```python
from build123d import *

# Parameters (mm, degrees)
AUFSATZ_LINEAR_AUSTRAGEN1_DEPTH             = 21
AUFSATZ_LINEAR_AUSTRAGEN1_DEPTH_BACK        = 21
SCHNITT_LINEAR_AUSTRAGEN1_DEPTH             = 35
SKIZZE9_R                                   = 4
SCHNITT_LINEAR_AUSTRAGEN2_DEPTH             = 21
SCHNITT_LINEAR_AUSTRAGEN3_REACH             = 35.5
SKIZZE11_R                                  = 3
SCHNITT_LINEAR_AUSTRAGEN3_DIRECTION_2_REACH = 35.5


with BuildPart() as part:
    # Skizze3 → Aufsatz-Linear austragen1 (new body, two sides)
    with BuildSketch(Plane.XY) as aufsatz_linear_austragen1_sk:
        Polygon((0, 205), (33.5, 205), (33.5, 130), (11, 130), (11, 155), (0, 155), (-11, 155), (-11, 130), (-33.5, 130), (-33.5, 205), align=None)
    extrude(amount=AUFSATZ_LINEAR_AUSTRAGEN1_DEPTH)
    extrude(aufsatz_linear_austragen1_sk.sketch, amount=-AUFSATZ_LINEAR_AUSTRAGEN1_DEPTH_BACK)

    # Skizze6 → Schnitt-Linear austragen1 (cut)
    with BuildSketch(Plane(origin=(0, 205, 0), x_dir=(1, 0, 0), z_dir=(0, 1, 0))):
        with BuildLine():
            Line((-25.25, 0), (-25.25, 21))
            Line((-25.25, 21), (33.5, 21))
            Line((33.5, 21), (33.5, -12.65))
            Line((33.5, -12.65), (-12.6, -12.65))
            ThreePointArc((-12.6, -12.65), (-21.544900782, -8.944900782), (-25.25, 0))
        make_face()
    extrude(amount=-SCHNITT_LINEAR_AUSTRAGEN1_DEPTH, mode=Mode.SUBTRACT)

    # Skizze9 → Schnitt-Linear austragen2 (cut)
    with BuildSketch(Plane.XY):
        with Locations((-13.5, 190)):
            Circle(SKIZZE9_R)
        with Locations((13.5, 190)):
            Circle(SKIZZE9_R)
    extrude(amount=SCHNITT_LINEAR_AUSTRAGEN2_DEPTH, mode=Mode.SUBTRACT)

    # Schnitt-Linear austragen3: up to this face of the body (flat: up to its plane)
    schnitt_linear_austragen3_end = Plane(part.part.faces().sort_by_distance((-33.5, 167.5, 0))[0])
    # Skizze11 → Schnitt-Linear austragen3 (cut, up to the picked face)
    with BuildSketch(Plane(origin=(0, 0, 0), x_dir=(0, 0, -1), z_dir=(1, 0, 0)), mode=Mode.PRIVATE) as schnitt_linear_austragen3_sk1:
        with Locations((7.5, 143)):
            Circle(SKIZZE11_R)
    schnitt_linear_austragen3_tool1 = split(extrude(schnitt_linear_austragen3_sk1.sketch, amount=-SCHNITT_LINEAR_AUSTRAGEN3_REACH, mode=Mode.PRIVATE), bisect_by=schnitt_linear_austragen3_end, keep=Keep.BOTH, mode=Mode.PRIVATE)
    add(schnitt_linear_austragen3_tool1.solids().sort_by_distance((0, 143, -7.5))[0], mode=Mode.SUBTRACT)
    # Skizze11 → Schnitt-Linear austragen3 (cut, up to the picked face)
    with BuildSketch(Plane(origin=(0, 0, 0), x_dir=(0, 0, -1), z_dir=(1, 0, 0)), mode=Mode.PRIVATE) as schnitt_linear_austragen3_sk2:
        with Locations((-7.5, 143)):
            Circle(SKIZZE11_R)
    schnitt_linear_austragen3_tool2 = split(extrude(schnitt_linear_austragen3_sk2.sketch, amount=-SCHNITT_LINEAR_AUSTRAGEN3_REACH, mode=Mode.PRIVATE), bisect_by=schnitt_linear_austragen3_end, keep=Keep.BOTH, mode=Mode.PRIVATE)
    add(schnitt_linear_austragen3_tool2.solids().sort_by_distance((0, 143, 7.5))[0], mode=Mode.SUBTRACT)

    # Schnitt-Linear austragen3 direction 2: up to this face of the body (flat: up to its plane)
    schnitt_linear_austragen3_direction_2_end = Plane(part.part.faces().sort_by_distance((33.5, 155.556787933, 2.493145519))[0])
    # Skizze11 → Schnitt-Linear austragen3 direction 2 (cut, up to the picked face)
    with BuildSketch(Plane(origin=(0, 0, 0), x_dir=(0, 0, -1), z_dir=(1, 0, 0)), mode=Mode.PRIVATE) as schnitt_linear_austragen3_direction_2_sk1:
        with Locations((7.5, 143)):
            Circle(SKIZZE11_R)
    schnitt_linear_austragen3_direction_2_tool1 = split(extrude(schnitt_linear_austragen3_direction_2_sk1.sketch, amount=SCHNITT_LINEAR_AUSTRAGEN3_DIRECTION_2_REACH, mode=Mode.PRIVATE), bisect_by=schnitt_linear_austragen3_direction_2_end, keep=Keep.BOTH, mode=Mode.PRIVATE)
    add(schnitt_linear_austragen3_direction_2_tool1.solids().sort_by_distance((0, 143, -7.5))[0], mode=Mode.SUBTRACT)
    # Skizze11 → Schnitt-Linear austragen3 direction 2 (cut, up to the picked face)
    with BuildSketch(Plane(origin=(0, 0, 0), x_dir=(0, 0, -1), z_dir=(1, 0, 0)), mode=Mode.PRIVATE) as schnitt_linear_austragen3_direction_2_sk2:
        with Locations((-7.5, 143)):
            Circle(SKIZZE11_R)
    schnitt_linear_austragen3_direction_2_tool2 = split(extrude(schnitt_linear_austragen3_direction_2_sk2.sketch, amount=SCHNITT_LINEAR_AUSTRAGEN3_DIRECTION_2_REACH, mode=Mode.PRIVATE), bisect_by=schnitt_linear_austragen3_direction_2_end, keep=Keep.BOTH, mode=Mode.PRIVATE)
    add(schnitt_linear_austragen3_direction_2_tool2.solids().sort_by_distance((0, 143, 7.5))[0], mode=Mode.SUBTRACT)


solid = part.part
```
Design review of the part built by this model. Coordinates are the model's own, in mm. A direction names the side the tool comes from. Give positions to 0.01 mm unless a question says otherwise; leave off trailing zeros. Write each loop counter-clockwise with the first axis right and the second up, starting at its lowest first coordinate (ties: lowest second). Pieces come first, ordered by that corner, then holes. Notation, with made-up numbers: (-11, 53.5) -> (8, 53.5) arc R20 ccw to (8, 84.5) -> close; hole circle Ø9 at (4.25, 41). An arc over 180 degrees is marked (long way). Answer in a Markdown table with one row per item.
(1) Consider section B-B (y = 190). State the section outline as (x, z) points.
Results:
| item | result |
|---|---|
| outline | (-33.5, -21) -> (-25.25, -21) -> (-25.25, 0) arc R12.65 cw to (-17.5, 11.66) -> (-17.5, 21) -> (-33.5, 21) -> close; (-9.5, 12.65) -> (9.5, 12.65) -> (9.5, 21) -> (-9.5, 21) -> close; (17.5, 12.65) -> (33.5, 12.65) -> (33.5, 21) -> (17.5, 21) -> close |
(2) Consider section A-A (x = 13.5). State the section outline as (y, z) points.
Results:
| item | result |
|---|---|
| outline | (130, -21) -> (170, -21) -> (170, 12.65) -> (186, 12.65) -> (186, 21) -> (130, 21) -> close; (194, 12.65) -> (205, 12.65) -> (205, 21) -> (194, 21) -> close; hole circle Ø6 at (143, -7.5); hole circle Ø6 at (143, 7.5) |
(3) For faces 1 (the flat face through (-22, 130, 0)), 2 (the flat face through (-25.25, 188, -10)), 3 (the flat face through (11, 142, 0)), list the 3-axis set-ups (+Z, -Z, +X, -X, +Y, -Y) from which the entire face can be reached by the end or side of a thin tool; tool diameter is ignored.
Results:
| item | result |
|---|---|
| face 1 | +Z, -Z, +X, -X, -Y |
| face 2 | -Z, +X, +Y |
| face 3 | +Z, -Z, -Y |
(4) Clearance check with flat-ended pins moving along their axes: pin 1 (9.5 mm diameter, centred on y = 143, z = -7.5, fed in from -X); pin 2 (6 mm diameter, centred on x = 1.5, z = 6.5, fed in from +Y); pin 3 (12 mm diameter, centred on x = 1.5, z = 13.5, fed in from -Y); pin 4 (8 mm diameter, centred on x = 18, y = 183.5, fed in from -Z). State where each tip first meets the part, or that it passes through.
Results:
| item | result |
|---|---|
| pin 1 | x = -33.5 |
| pin 2 | y = 170 |
| pin 3 | y = 155 |
| pin 4 | z = 12.65 |
(5) Consider section C-C (z = -1). State the section outline as (x, y) points.
Results:
| item | result |
|---|---|
| outline | (-33.5, 130) -> (-11, 130) -> (-11, 155) -> (11, 155) -> (11, 130) -> (33.5, 130) -> (33.5, 170) -> (-25.25, 170) -> (-25.25, 205) -> (-33.5, 205) -> close |
(6) To check wall thickness, follow probe 1 along Z at (x, y) = (-20.25, 143); probe 2 along X at (y, z) = (190, 15); probe 3 along Y at (x, z) = (22, 7.5). State the ranges of each line that lie inside material, in increasing order.
Results:
| item | result |
|---|---|
| probe 1 | -21 to -10.5, -4.5 to 4.5, 10.5 to 21 |
| probe 2 | -33.5 to -17.5, -9.5 to 9.5, 17.5 to 33.5 |
| probe 3 | 130 to 140, 146 to 170 |
(7) Consider section D-D (y = 143). State the section outline as (x, z) points, then the cut area to 3 significant figures.
Results:
| item | result |
|---|---|
| outline | (-33.5, -21) -> (-11, -21) -> (-11, -10.5) -> (-33.5, -10.5) -> close; (-33.5, -4.5) -> (-11, -4.5) -> (-11, 4.5) -> (-33.5, 4.5) -> close; (-33.5, 10.5) -> (-11, 10.5) -> (-11, 21) -> (-33.5, 21) -> close; (11, -21) -> (33.5, -21) -> (33.5, -10.5) -> (11, -10.5) -> close; (11, -4.5) -> (33.5, -4.5) -> (33.5, 4.5) -> (11, 4.5) -> close; (11, 10.5) -> (33.5, 10.5) -> (33.5, 21) -> (11, 21) -> close |
| area | 1,350 mm2 |
(8) Mouldability with a two-part tool opening along Z and no side actions: class faces 4 (the flat face through (0, 155, 0)), 5 (the cylindrical face through (22.09, 145.53, -9.11)), 6 (the flat face through (11, 184, 12.65)) as +Z half, -Z half, draft (parallel to the pull), parting line (faces both ways), or undercut.
Results:
| item | result |
|---|---|
| face 4 | draft |
| face 5 | undercut |
| face 6 | -Z half |
